Autodesk Inventor part; units mm, degrees
ref_plane "YZ Plane" through (0, 0, 0) normal (1, 0, 0) x (0, 1, 0)
ref_plane "XZ Plane" through (0, 0, 0) normal (0, 1, 0) x (-1, 0, 0)
ref_plane "XY Plane" through (0, 0, 0) normal (0, 0, 1) x (1, 0, 0)
sketch "Sketch1" plane through (0, 0, 0) normal (0, 1, 0) x (-1, 0, 0)
  line L0 (-15, 15) -> (15, 15)
  line L1 (15, 15) -> (15, -15)
  line L2 (15, -15) -> (-15, -15)
  line L3 (-15, -15) -> (-15, 15)
  line L4 (-15, 15) -> (15, -15) construction
  line L5 (15, 15) -> (-15, -15) construction
  line L6 (21, 0) -> (-21, 0) construction
  line L7 (0, -21) -> (0, 21) construction
  line L8 (0, 8) -> (0, 0) construction
  line L9 (-3.4, 8) -> (-3.4, 0)
  line L10 (3.4, 0) -> (3.4, 8)
  arc A0 (3.4, 8) -> (-3.4, 8) centre (0, 8) ccw
  arc A1 (-3.4, 0) -> (3.4, 0) centre (0, 0) ccw
  point P0 (0, 0)
  point P1 (0, 4)
  point P2 (10, 0)
  point P3 (-10, 0)
  point P4 (0, 4)
  dimension "d0" = 30
  dimension "d1" = 30
  dimension "d2" = 6.8
  dimension "d3" = 8
  dimension "d4" = 0
  dimension "d5" = 20
extrude "Extrusion1" add sketch "Sketch1" against normal blind 12 contours L0 L1 L2 L3 | A0 L10 A1 L9
extrude "Extrusion2" cut sketch "Sketch1" against normal blind 8
hole "Hole1" at (0, 0, 4) direction (0, -1, 0) diameter 4.917 end through all countersink diameter 6 countersink angle 90
sketch "Sketch2" plane through (0, -8, 0) normal (0, 1, 0) x (1, 0, 0)
  point P0 (0, 0)
  point P1 (10, 0)
  point P2 (-10, 0)
hole "Hole2" at (10, -8, 0) at (-10, -8, 0) direction (0, -1, 0) diameter 4 end through all countersink diameter 9 countersink angle 90
fillet "Fillet1" radius 5 4 edges at (-15, -10, -15) (-15, -10, 15) (15, -10, 15) (15, -10, -15)
properties part number "TCSM1-004" material "Steel"
The model under review builds one solid part; all positions refer to its coordinate system, in mm. A direction names the side the tool comes from. Round coordinates to 2 decimals unless told otherwise and drop trailing zeros. Loops run counter-clockwise (first coordinate to the right, second up) from the corner with the lowest first, then second, coordinate; pieces in that order, holes last. Notation, with made-up numbers: (-4.75, 1.25) -> (47.25, 1.25) arc R28 ccw to (47.25, 34.25) -> close; hole circle Ø6 at (65.5, 60). An arc over 180 degrees is marked (long way). Write item = value, one per line. Start each with the question number.
Item 1: For faces 1 (the cylindrical face through (-0.1, -3.9, 11.4)), 2 (the flat face through (-3.4, -4, 4)), 3 (the conical face through (-8.54, -10.34, -1.59)), list the 3-axis set-ups (+Z, -Z, +X, -X, +Y, -Y) from which the entire face can be reached by the end or side of a thin tool; tool diameter is ignored.
Item 2: Take a section at B-B on x = 0. Give the boundary of the cut face in (y, z).
Item 3: Mouldability with a two-part tool opening along Z and no side actions: class faces 4 (the cylindrical face through (-0.738, -6.351, 6.345)), 5 (the cylindrical face through (0.1, -3.9, -3.4)), 6 (the flat face through (0, 0, 0.8)), 7 (the cylindrical face through (8, -11, 0)) as released by +Z, released by -Z, zero draft, split by the parting line, or undercut.
Item 4: Insertion check: pin 1 (3 mm diameter, centred on x = 0, z = 4, fed in from +Y); pin 2 (3 mm diameter, centred on y = -6, z = 1, fed in from +X); pin 3 (3 mm diameter, centred on x = -8.5, z = 6, fed in from +Y). Each pin has a flat end and moves straight along its axis. Give the tip position at first contact, or say it passes through.
Item 5: To check wall thickness, follow L1, parallel to X at y = -11.1, z = 0; L2, parallel to Z at x = -10, y = -11.55; L3, parallel to Z at x = 0, y = -4.5. State the ranges of each line that lie inside material, in increasing order.
Item 6: Take a section at A-A on y = -9.5. Give the boundary of the cut face in (x, z), plus the area to 3 significant figures.
Item 7: Take a section at D-D on z = -6. Give the boundary of the cut face in (x, y), plus the area to 3 significant figures.
Item 8: Take a section at C-C on y = -4.75. Give the boundary of the cut face in (x, z), plus the area to 3 significant figures.
Result:
q1.face_1 = +Z, +Y
q1.face_2 = +Z, -Z, -X, +Y
q1.face_3 = +Y
q2.outline = (-12, -15) -> (-8, -15) -> (-8, -3.4) -> (0, -3.4) -> (0, 1) -> (-0.54, 1.54) -> (-12, 1.54) -> close; (-12, 6.46) -> (-0.54, 6.46) -> (0, 7) -> (0, 11.4) -> (-8, 11.4) -> (-8, 15) -> (-12, 15) -> close
q3.face_4 = undercut
q3.face_5 = released by -Z
q3.face_6 = zero draft
q3.face_7 = undercut
q4.pin_1 = through
q4.pin_2 = 3.4
q4.pin_3 = -8
q5.L1 = -15 to -12, -8 to 8, 12 to 15
q5.L2 = -15 to -2, 2 to 15
q5.L3 = -3.4 to 1.54, 6.46 to 11.4
q6.outline = (-15, -10) arc R5 ccw to (-10, -15) -> (10, -15) arc R5 ccw to (15, -10) -> (15, 10) arc R5 ccw to (10, 15) -> (-10, 15) arc R5 ccw to (-15, 10) -> close; hole circle Ø6 at (-10, 0); hole circle Ø4.92 at (0, 4); hole circle Ø6 at (10, 0)
q6.area = 803 mm²
q7.outline = (-15, -12) -> (15, -12) -> (15, -8) -> (-15, -8) -> close
q7.area = 120 mm²
q8.outline = (-3.4, 0) arc R3.4 ccw to (3.4, 0) -> (3.4, 8) arc R3.4 ccw to (-3.4, 8) -> close; hole circle Ø4.92 at (0, 4)
q8.area = 71.7 mm²
